```python
from build123d import *

# Parameters (mm, degrees)
BOSS_EXTRUDE1_DEPTH = 20
FILLET1_R           = 1.5
SKETCH2_R           = 7
SKETCH2_R_2         = 2.25
CUT_EXTRUDE1_DEPTH  = 1
SKETCH3_R           = 1.5
CUT_EXTRUDE2_DEPTH  = 3


with BuildPart() as part:
    # Sketch1 → Boss-Extrude1 (new body)
    with BuildSketch(Plane.XY):
        with BuildLine():
            Line((-33, 12.5), (33, 12.5))
            ThreePointArc((33, 12.5), (45.5, 0), (33, -12.5))
            Line((33, -12.5), (-33, -12.5))
            ThreePointArc((-33, -12.5), (-45.5, 0), (-33, 12.5))
        make_face()
    extrude(amount=BOSS_EXTRUDE1_DEPTH)

    # Fillet1
    fillet1_edges = [part.edges().sort_by_distance(p)[0] for p in [
        (-45.5, 0, 20),
        (0, -12.5, 20),
        (45.5, 0, 20),
        (0, -12.5, 0),
        (-45.5, 0, 0),
        (0, 12.5, 0),
        (45.5, 0, 0),
        (0, 12.5, 20),
    ]]
    fillet(fillet1_edges, radius=FILLET1_R)

    # Sketch2 → Cut-Extrude1 (cut)
    with BuildSketch(Plane.XY.offset(20)):
        with Locations((-22.5, 0)):
            Circle(SKETCH2_R)
        with Locations((22.5, 0)):
            Circle(SKETCH2_R)
        Circle(SKETCH2_R_2)
    extrude(amount=-CUT_EXTRUDE1_DEPTH, mode=Mode.SUBTRACT)

    # Sketch3 → Cut-Extrude2 (cut)
    with BuildSketch(Plane.XZ.offset(12.5)):
        with Locations(Location((-17.5, 10, 0), (0, 0, 270))):
            Circle(SKETCH3_R)
        with Locations(Location((16.5, 10, 0), (0, 0, 90))):
            Circle(SKETCH3_R)
    extrude(amount=-CUT_EXTRUDE2_DEPTH, mode=Mode.SUBTRACT)


solid = part.part
```
Here's how the part is built. I have some questions about the finished solid (model axes, mm). A direction names the side the tool comes from. Coordinates: 2 decimals unless noted, no trailing zeros. Loops run counter-clockwise (first coordinate to the right, second up) from the corner with the lowest first, then second, coordinate; pieces in that order, holes last. Notation, with made-up numbers: M -7.5,66.25 L 25.5,66.25 A15 ccw 25.5,80.25 Z; hole C -8,12 d11. An arc over 180 degrees is marked long. One line per item, written item: value.
1. Please list where these lines run through material, in increasing order: probe 1 along X at (y, z) = (-10.9, 10); probe 2 along X at (y, z) = (-10.6, 10); probe 3 along Z at (x, y) = (-23, -6).
Geometry says:
probe 1: x = -39.12 to -19, -16 to 15, 18 to 39.12
probe 2: x = -39.62 to -19, -16 to 15, 18 to 39.62
probe 3: z = 0 to 19
2. Imagine slicing it at C-C (z = 10). List the corners of the cut face in (x, y) for me.
Geometry says:
outline: M -33,-12.5 L -19,-12.5 L -19,-9.5 L -16,-9.5 L -16,-12.5 L 15,-12.5 L 15,-9.5 L 18,-9.5 L 18,-12.5 L 33,-12.5 A12.5 ccw 33,12.5 L -33,12.5 A12.5 ccw Z
3. Thinking about a two-plate mould opening in Z: for faces 1 (the cylindrical face through (16.43, -11.02, 8.5)), 2 (the flat face through (1, 3, 20)), 3 (the flat face through (1, 0, 0)), which applies, +Z half, -Z half, draft (parallel to the pull), parting line (faces both ways), or undercut?
Geometry says:
face 1: undercut
face 2: +Z half
face 3: -Z half
4. Imagine slicing it at D-D (x = -17.5). List the corners of the cut face in (y, z) for me.
Geometry says:
outline: M -12.5,1.5 A1.5 ccw -11,0 L 11,0 A1.5 ccw 12.5,1.5 L 12.5,18.5 A1.5 ccw 11,20 L 4.9,20 L 4.9,19 L -4.9,19 L -4.9,20 L -11,20 A1.5 ccw -12.5,18.5 L -12.5,11.5 L -9.5,11.5 L -9.5,8.5 L -12.5,8.5 Z
5. Will these pins go through, and if not, where does the flat tip stop? pin 1 Ø0.9 at (x, z) = (16, 10.5) entering from -Y; pin 2 Ø4 at (x, y) = (0, 0) entering from +Z; pin 3 Ø1.5 at (y, z) = (-8.5, 7.5) entering from +X.
Geometry says:
pin 1: stops at y = -9.5
pin 2: stops at z = 19
pin 3: stops at x = 42.81
6. On a 3-axis mill with a long thin cutter (end or side, diameter ignored), from which of +Z, -Z, +X, -X, +Y, -Y can I reach the whole of each face in a straight line? I mean faces 4 (the cylindrical face through (-16.49, -11.02, 11.11)), 5 (the flat face through (0, 0, 19)), 6 (the flat face through (0, 12.5, 10)). Say none if no direction works.
Geometry says:
face 4: -Y
face 5: +Z
face 6: +Z, -Z, +X, -X, +Y
7. Imagine slicing it at B-B (x = 22.5). List the corners of the cut face in (y, z) for me, and give its area (3 significant figures).
Geometry says:
outline: M -12.5,1.5 A1.5 ccw -11,0 L 11,0 A1.5 ccw 12.5,1.5 L 12.5,18.5 A1.5 ccw 11,20 L 7,20 L 7,19 L -7,19 L -7,20 L -11,20 A1.5 ccw -12.5,18.5 Z
area: 484 mm2
8. Imagine slicing it at A-A (y = 0). List the corners of the cut face in (x, z) for me, and give its area (3 significant figures).
Geometry says:
outline: M -45.5,1.5 A1.5 ccw -44,0 L 44,0 A1.5 ccw 45.5,1.5 L 45.5,18.5 A1.5 ccw 44,20 L 29.5,20 L 29.5,19 L 15.5,19 L 15.5,20 L 2.25,20 L 2.25,19 L -2.25,19 L -2.25,20 L -15.5,20 L -15.5,19 L -29.5,19 L -29.5,20 L -44,20 A1.5 ccw -45.5,18.5 Z
area: 1,790 mm2
